```python
from build123d import *

# Parameters (mm, degrees)
BOSS_EXTRUDE1_DEPTH     = 10
CUT_EXTRUDE1_DEPTH      = 30
CUT_EXTRUDE1_DEPTH_BACK = 30
CUT_EXTRUDE4_DEPTH      = 8.25
CUT_EXTRUDE4_DEPTH_BACK = 8.25
FILLET3_R               = 0.5
BOSS_EXTRUDE2_START     = -6
SKETCH4_W               = 15
SKETCH4_H               = 25
BOSS_EXTRUDE2_DEPTH     = 2
FILLET5_R               = 6
FILLET10_R              = 2
FILLET19_R              = 6
SKETCH9_W               = 1.113670972
SKETCH9_H               = 16.5
CUT_EXTRUDE5_DEPTH      = 10
FILLET21_R              = 1


with BuildPart() as part:
    # Sketch1 → Boss-Extrude1 (new body)
    with BuildSketch(Plane.XY):
        Polygon((-6, -21), (6, -21), (6, 21), (-6, 21), (-6, 8.25), (-2, 8.25), (-2, -8.25), (-6, -8.25), align=None)
    extrude(amount=BOSS_EXTRUDE1_DEPTH)

    # Sketch2 → Cut-Extrude1 (cut, two sides: drawn at the far end of the back side and taken through both)
    with BuildSketch(Plane(origin=(0, 0, 0), x_dir=(1, 0, 0), z_dir=(0, 1, 0)).offset(-CUT_EXTRUDE1_DEPTH_BACK)):
        Polygon((-2, -10), (6, -5), (6, -10), align=None)
    extrude(amount=CUT_EXTRUDE1_DEPTH + CUT_EXTRUDE1_DEPTH_BACK, mode=Mode.SUBTRACT)

    # Sketch8 → Cut-Extrude4 (cut, two sides: drawn at the far end of the back side and taken through both)
    with BuildSketch(Plane(origin=(0, 0, 0), x_dir=(1, 0, 0), z_dir=(0, 1, 0)).offset(-CUT_EXTRUDE4_DEPTH_BACK)):
        Polygon((-2, 0), (-2, -9), (5, -4.466137359), (5, 0), align=None)
    extrude(amount=CUT_EXTRUDE4_DEPTH + CUT_EXTRUDE4_DEPTH_BACK, mode=Mode.SUBTRACT)

    # Fillet3
    fillet3_edges = [part.edges().sort_by_distance(p)[0] for p in [
        (-6, 14.625, 10),
        (6, 0, 0),
        (-6, -14.625, 10),
    ]]
    fillet(fillet3_edges, radius=FILLET3_R)

    # Sketch4 → Boss-Extrude2 (add)
    with BuildSketch(Plane(origin=(0, 0, 0), x_dir=(0, 0, -1), z_dir=(1, 0, 0)).offset(BOSS_EXTRUDE2_START)):
        with Locations((7.5, 0)):
            Rectangle(SKETCH4_W, SKETCH4_H)
    extrude(amount=BOSS_EXTRUDE2_DEPTH)

    # Fillet5
    fillet5_edges = [part.edges().sort_by_distance(p)[0] for p in [
        (-4, -10.375, 0),
        (-4, 10.375, 0),
    ]]
    fillet(fillet5_edges, radius=FILLET5_R)

    # Fillet10
    fillet10_edges = [part.edges().sort_by_distance(p)[0] for p in [
        (-2, 12.5, 0),
        (-2, -12.5, 0),
    ]]
    fillet(fillet10_edges, radius=FILLET10_R)

    # Fillet19
    fillet19_edges = [part.edges().sort_by_distance(p)[0] for p in [
        (6, 0, 5),
    ]]
    fillet(fillet19_edges, radius=FILLET19_R)

    # Sketch9 → Cut-Extrude5 (cut)
    with BuildSketch(Plane.XY):
        with Locations((-2, 0)):
            Rectangle(SKETCH9_W, SKETCH9_H)
    extrude(amount=CUT_EXTRUDE5_DEPTH, mode=Mode.SUBTRACT)

    # Fillet21
    # the kernel refuses this fillet: 1 mm, written as the material it adds along each edge
    with BuildSketch(Plane(origin=(5, -9.609341418, 4.466137359), x_dir=(0, 0, -1), z_dir=(0, 1, 0))) as fillet21_piece_1:
        with BuildLine():
            CenterArc((FILLET21_R * 0.543736567297, FILLET21_R), FILLET21_R, 212.930914829, 57.069085171)
            Line((-FILLET21_R * 0.295590096809, FILLET21_R * 0.456372599182), (0, 0))
            Line((0, 0), (FILLET21_R * 0.543736567297, 0))
        make_face()
    extrude(amount=19.218682836)
    # the kernel refuses this fillet: 1 mm, written as the material it takes off along each edge
    with BuildSketch(Plane(origin=(5, 8.25, 0), x_dir=(1, 0, 0), z_dir=(0, -1, 0))) as fillet21_2_piece_1:
        with BuildLine():
            CenterArc((FILLET21_R, FILLET21_R), FILLET21_R, 180, 90)
            Line((0, FILLET21_R), (0, 0))
            Line((0, 0), (FILLET21_R, 0))
        make_face()
    extrude(amount=16.5, mode=Mode.SUBTRACT)
    with BuildSketch(Plane(origin=(-1.443164514, -8.25, 8.639340628), x_dir=(0, 0, 1), z_dir=(0, 1, 0))) as fillet21_2_piece_2:
        with BuildLine():
            CenterArc((FILLET21_R * 0.543736567297, FILLET21_R), FILLET21_R, 212.930914829, 57.069085171)
            Line((-FILLET21_R * 0.295590096809, FILLET21_R * 0.456372599182), (0, 0))
            Line((0, 0), (FILLET21_R * 0.543736567297, 0))
        make_face()
    extrude(amount=16.5, mode=Mode.SUBTRACT)
    with BuildSketch(Plane(origin=(-1.443164514, -8.25, 9.651977821), x_dir=(0.8479983040050877, 0, -0.5299989400031806), z_dir=(0, 1, 0))) as fillet21_2_piece_3:
        with BuildLine():
            CenterArc((FILLET21_R * 1.80424764151, FILLET21_R), FILLET21_R, 147.994616792, 122.005383208)
            Line((FILLET21_R * 0.956249337502, FILLET21_R * 1.52999894), (0, 0))
            Line((0, 0), (FILLET21_R * 1.80424764151, 0))
        make_face()
    extrude(amount=16.5, mode=Mode.SUBTRACT)


solid = part.part
```
Could you check a few things on this model? Use its own coordinates, in mm. A direction names the side the tool comes from. Coordinates: 2 decimals unless noted, no trailing zeros. Order: outer loops, then holes, each group sorted by start corner. A loop starts at its lowest first (then second) coordinate and runs counter-clockwise, first axis right, second up. Notation, with made-up numbers: M -33,-6 L 2,-6 A13 cw 2,10 Z; hole C 83.25,70 d8. An arc over 180 degrees is marked long. Use a Markdown table: item, result. Add a question column.
Q1. Which directions (+Z, -Z, +X, -X, +Y, -Y) give clear straight access to the entire face, cutting with the end or side of a thin tool? Please do faces 4 (the cylindrical face through (-0.593, -0.116, 8.836)), 5 (the flat face through (-5, -12.5, -8)), 6 (the flat face through (1, -16, 0)).
Q2. I want a section at B-B on x = -4.75. List the corners of the cut face in (y, z) for me.
Q3. I want a section at D-D on z = -1. List the corners of the cut face in (x, y) for me.
Q4. If I drill on L1, parallel to Y at x = 4.25, z = 2; L2, parallel to Z at x = -3.5, y = -18.5; L3, parallel to X at y = -11, z = -9.25, over which ranges is the centre line in solid material (lowest first)?
Q5. I'm going to push flat-ended pins straight in: pin 1 (2 mm diameter, centred on x = -5.5, y = -3, fed in from +Z); pin 2 (3 mm diameter, centred on y = -11.5, z = -7, fed in from +X); pin 3 (3 mm diameter, centred on y = 1.5, z = 3, fed in from -X); pin 4 (1.5 mm diameter, centred on x = 0.5, z = -2.5, fed in from +Y). Where does each tip first touch, or does it pass through?
Q6. We'd pull the mould along Y, two halves only. Please class faces 1 (the flat face through (-5, 0, 0)), 2 (the flat face through (-5, 12.5, -8)), 3 (the flat face through (6, 0, 1)): pulls with the +Y half, pulls with the -Y half, needs draft (parallel to the pull), parting line crosses it, or undercut.
Q7. I want a section at C-C on y = -15.5. List the corners of the cut face in (x, z) for me, then the cut area to 3 significant figures.
Q8. I want a section at A-A on y = -5. List the corners of the cut face in (x, z) for me.
Checked values:
| question | item | result |
|---|---|---|
| 1 | face 4 | +Z |
| 1 | face 5 | -Z, +X, -X, -Y |
| 1 | face 6 | -Z, +X, -Y |
| 2 | outline | M -21,0 L -14.5,0 A2 cw -12.5,-2 L -12.5,-15 L 12.5,-15 L 12.5,-2 A2 cw 14.5,0 L 21,0 L 21,10 L 8.25,10 L 8.25,0 L -8.25,0 L -8.25,10 L -21,10 Z |
| 3 | outline | M -6,-12.77 L -1.32,-12.77 L -1.32,-8.25 L -4,-8.25 L -4,8.25 L -1.32,8.25 L -1.32,12.77 L -6,12.77 Z |
| 4 | L1 | -21 to -8.25, 8.25 to 21 |
| 4 | L2 | 0 to 10 |
| 4 | L3 | -6 to -4 |
| 5 | pin 1 | z = 0 |
| 5 | pin 2 | x = -3.98 |
| 5 | pin 3 | x = 4.82 |
| 5 | pin 4 | through |
| 6 | face 1 | undercut |
| 6 | face 2 | pulls with the +Y half |
| 6 | face 3 | needs draft |
| 7 | outline | M -6,0 L 5.5,0 A0.5 ccw 6,0.5 L 6,1.67 A6 ccw 3.18,6.76 L -2,10 L -5.5,10 A0.5 ccw -6,9.5 Z |
| 7 | area | 98.2 mm² |
| 8 | outline | M -6,-15 L -4,-15 L -4,0 L -6,0 Z; M -1.19,8.52 A1 ccw -0.99,8.34 L 4.54,4.76 A1 cw 5,3.92 L 5,1 A1 ccw 5.71,0.04 A0.5 ccw 6,0.5 L 6,1.67 A6 ccw 3.18,6.76 L 0.09,8.7 A1 ccw Z |
